Autodesk Inventor part; units mm, degrees
ref_plane "YZ Plane" through (0, 0, 0) normal (1, 0, 0) x (0, 1, 0)
ref_plane "XZ Plane" through (0, 0, 0) normal (0, 1, 0) x (-1, 0, 0)
ref_plane "XY Plane" through (0, 0, 0) normal (0, 0, 1) x (1, 0, 0)
sketch "Sketch1" plane through (0, 0, 0) normal (0, 0, 1) x (1, 0, 0)
  line L0 (0, 0) -> (-56.9976, 0)
  line L1 (-56.9976, 50.8) -> (0, 50.8)
  line L2 (0, 50.8) -> (-7.493, 50.8)
  line L3 (-7.493, 50.8) -> (-7.493, 44.45)
  line L4 (-56.9976, 50.8) -> (-49.5046, 50.8)
  line L5 (-49.5046, 50.8) -> (-49.5046, 44.45)
  circle A0 centre (-49.5046, 44.45) radius 3.302
  circle A1 centre (-7.493, 44.45) radius 3.302
  circle A2 centre (-62.865, 14.1224) radius 3.2004
  circle A3 centre (5.8801, 14.1224) radius 3.2004
  line L6 (-56.9976, 50.8) -> (-69.6976, 50.8)
  line L7 (-69.6976, 50.8) -> (-69.6976, 0)
  line L8 (-69.6976, 0) -> (-56.9976, 0)
  line L9 (0, 50.8) -> (8.89, 50.8)
  line L10 (8.89, 0) -> (0, 0)
  line L11 (0, 50.8) -> (12.7, 50.8)
  line L12 (12.7, 50.8) -> (12.7, 0)
  line L13 (12.7, 0) -> (0, 0)
  dimension "d1" = 56.9976
  dimension "d2" = 50.8
  dimension "d3" = 7.493
  dimension "d4" = 6.35
  dimension "d5" = 7.493
  dimension "d6" = 6.604
  dimension "d7" = 6.604
  dimension "d19" = 6.35
  dimension "d46" = 6.4008
  dimension "d47" = 6.4008
  dimension "d48" = 12.7
  dimension "d51" = 50.8
  dimension "d53" = 36.6776
  dimension "d55" = 36.6776
  dimension "d57" = 12.7
  dimension "d58" = 6.8199
  dimension "d59" = 6.8326
extrude "Plate5" add sketch "Sketch1" along normal blind 3.175
equation "\"BendRadius\" = Thickness"
equation "\"BendReliefWidth\" = Thickness"
equation "\"BendReliefDepth\" = 0.5 * Thickness"
equation "\"CornerReliefSize\" = 4 * Thickness"
equation "\"MinimumRemnant\" = 2 * Thickness"
equation "\"TransitionRadius\" = BendRadius"
equation "\"JacobiRadiusSize\" = BendRadius"
equation "\"GapSize\" = Thickness"
equation "\"d8\" = BendRadius"
equation "\"d56\" = BendRadius"
properties part number "face mount" material "Aluminum 6061"
Source: CAD feature listing. Evaluate the final solid. Frame: model axes, mm. Round coordinates to 2 decimals unless told otherwise and drop trailing zeros. Loops run counter-clockwise (first coordinate to the right, second up) from the corner with the lowest first, then second, coordinate; pieces in that order, holes last. Notation, with made-up numbers: (52, 40.5) -> (105, 40.5) arc R17 cw to (105, 46.5) -> close; hole circle Ø4 at (80, -29.5). An arc over 180 degrees is marked (long way). Answer as a JSON object with one key per item and string values. Group by question number.
Q1. Section query A-A (y = 44.45). Output: boundary loops of the cut face in (x, z) (3 decimals), plus the area to 3 significant figures.
Q2. Contact query for a flat-ended pin moving along its axis: P1, Ø6, axis at x = -25, y = 34.5, coming from the -Z side. Output: stop coordinate, or through.
Q3. Section query D-D (x = 3.5). Output: boundary loops of the cut face in (y, z) (3 decimals), plus the area to 3 significant figures.
Q4. Mould query, pull axis X, two halves, no side actions, for faces 1 (the flat face through (12.7, 26, 2)), 2 (the cylindrical face through (-59.8, 13.2, 1.6)), 3 (the flat face through (-29, 26, 3.175)). Classes: pulls with the +X half, pulls with the -X half, needs draft (parallel to the pull), parting line crosses it, or undercut.
Q5. Ray query, line 1 (X direction, y = 44.5, z = 1.85); line 2 (X direction, y = 41.5, z = 2.1); line 3 (Y direction, x = -65, z = 2.05). Return the intervals inside material, ascending. Write a range as from..to.
Q6. Section query B-B (x = -47). Output: boundary loops of the cut face in (y, z) (3 decimals).
Q7. Section query C-C (z = 1.7). State how many separate pieces and enclosed holes the cut face has, plus the area to 3 significant figures.
Completed:
{
 "1": {"outline": "(-69.698, 0) -> (-52.807, 0) -> (-52.807, 3.175) -> (-69.698, 3.175) -> close; (-46.203, 0) -> (-10.795, 0) -> (-10.795, 3.175) -> (-46.203, 3.175) -> close; (-4.191, 0) -> (12.7, 0) -> (12.7, 3.175) -> (-4.191, 3.175) -> close", "area": "220 mm²"},
 "2": {"P1": "z = 0"},
 "3": {"outline": "(0, 0) -> (11.983, 0) -> (11.983, 3.175) -> (0, 3.175) -> close; (16.262, 0) -> (50.8, 0) -> (50.8, 3.175) -> (16.262, 3.175) -> close", "area": "148 mm²"},
 "4": {"face 1": "pulls with the +X half", "face 2": "undercut", "face 3": "needs draft"},
 "5": {"line 1": "-69.7..-52.81, -46.2..-10.79, -4.19..12.7", "line 2": "-69.7..-50.99, -48.02..-8.98, -6.01..12.7", "line 3": "0..11.74, 16.51..50.8"},
 "6": {"outline": "(0, 0) -> (42.298, 0) -> (42.298, 3.175) -> (0, 3.175) -> close; (46.602, 0) -> (50.8, 0) -> (50.8, 3.175) -> (46.602, 3.175) -> close"},
 "7": {"separate pieces": "1", "enclosed holes": "4", "area": "4,050 mm²"}
}
